Autodesk Inventor part; units mm, degrees
ref_plane "YZ Plane" through (0, 0, 0) normal (1, 0, 0) x (0, 1, 0)
ref_plane "XZ Plane" through (0, 0, 0) normal (0, 1, 0) x (-1, 0, 0)
ref_plane "XY Plane" through (0, 0, 0) normal (0, 0, 1) x (1, 0, 0)
sketch "スケッチ1" plane through (0, 0, 0) normal (0, 0, 1) x (1, 0, 0)
  circle A0 centre (0, 0) radius 1.5
  line L0 (-2.8284, 0) -> (0, 2.8284)
  line L1 (0, 2.8284) -> (2.8284, 0)
  line L2 (2.8284, 0) -> (0, -2.8284)
  line L3 (0, -2.8284) -> (-2.8284, 0)
  dimension "d0" = 3
  dimension "d1" = 4
extrude "押し出し1" add sketch "スケッチ1" against normal blind 420
properties part number "MainRod" material "CFRP"
Geometry check sheet. Reference: the model listing, model coordinates, mm. Coordinates: 2 decimals unless noted, no trailing zeros. Write each loop counter-clockwise with the first axis right and the second up, starting at its lowest first coordinate (ties: lowest second). Pieces come first, ordered by that corner, then holes. Notation, with made-up numbers: (75.25, 69.25) -> (87.25, 69.25) arc R18 ccw to (87.25, 78.25) -> close; hole circle Ø2 at (84, -16). An arc over 180 degrees is marked (long way). One line per question, with ' | ' between items.
1. Depth check by flat-ended pin: pin 1 Ø1.5 at (x, z) = (-2, -155.5) entering from -Y; pin 2 Ø1.5 at (y, z) = (1, -214) entering from -X; pin 3 Ø1.5 at (x, z) = (0.5, -81.5) entering from -Y. Enter the tip coordinate at first touch or a pass-through.
Answers:
pin 1: stops at y = -1.58 | pin 2: stops at x = -2.58 | pin 3: stops at y = -2.83
2. Cross-section at A-A on z = -380. Record the cut outline in (x, y), and give its area (3 significant figures).
Answers:
outline: (-2.83, 0) -> (0, -2.83) -> (2.83, 0) -> (0, 2.83) -> close; hole circle Ø3 at (0, 0) | area: 8.93 mm²
3. Thickness scan on probe 1 along Y at (x, z) = (0, -172); probe 2 along Y at (x, z) = (-0.35, -133); probe 3 along X at (y, z) = (1.2, -177.5). Record the ranges inside material, lowest first. Write a range as from..to.
Answers:
probe 1: y = -2.83..-1.5, 1.5..2.83 | probe 2: y = -2.48..-1.46, 1.46..2.48 | probe 3: x = -1.63..-0.9, 0.9..1.63
